Answer from the drawing. Dimensions are ordinates in mm from the lowest x, y and z of the part. Round coordinates to 2 decimals unless told otherwise and drop trailing zeros. Loops run counter-clockwise (first coordinate to the right, second up) from the corner with the lowest first, then second, coordinate; pieces in that order, holes last. Notation, with made-up numbers: (81, -14.75) - (92, -14.75) arc R17 cw to (92, 16.25) - close; hole circle Ø2 at (-30, 80). An arc over 180 degrees is marked (long way). Answer as CSV lines item,"result". Start each with the question number.
Q1. Each of these flat-tipped pins is pushed along its axis until it touches: pin 1 Ø9 at (x, z) = (11, 8.5) entering from -Y; pin 2 Ø8 at (x, y) = (17, 24.5) entering from -Z; pin 3 Ø5 at (x, y) = (21, 23.5) entering from +Z. Where does it stop, or does it pass through?
Q2. Section A-A on x = 12.25 is taken. Write down the section's boundary in (y, z).
Q3. Section B-B on y = 6 is taken. Write down the section's boundary in (x, z), then the cut area to 3 significant figures.
Q4. A straight line is drawn through the part: L1, parallel to Z at x = 20.25, y = 22. Find the intervals that lie inside material, in ascending order. Write a range as [from, to].
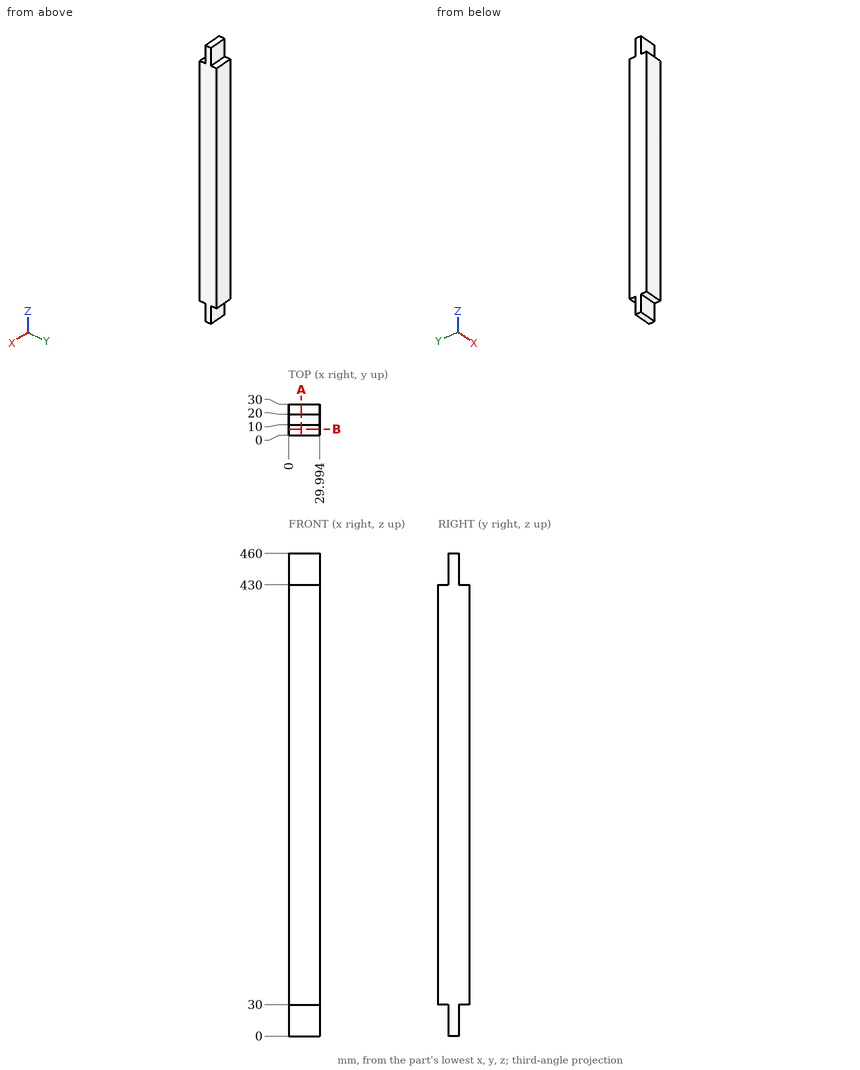
Findings:
1,pin 1,"stops at y = 10"
1,pin 2,"stops at z = 30"
1,pin 3,"stops at z = 430"
2,outline,"(0, 30) - (10, 30) - (10, 0) - (20, 0) - (20, 30) - (30, 30) - (30, 430) - (20, 430) - (20, 460) - (10, 460) - (10, 430) - (0, 430) - close"
3,outline,"(0, 30) - (29.99, 30) - (29.99, 430) - (0, 430) - close"
3,area,"12,000 mm^2"
4,L1,"z = [30, 430]"
